Model file for the job. Use its own axes, mm. A direction names the side the tool comes from. Round coordinates to 2 decimals unless told otherwise and drop trailing zeros. Loops run counter-clockwise (first coordinate to the right, second up) from the corner with the lowest first, then second, coordinate; pieces in that order, holes last. Notation, with made-up numbers: M 80.25,0 L 92.25,0 A29 ccw 92.25,21 Z; hole C -37,56.5 d10. An arc over 180 degrees is marked long. Use a Markdown table: item, result. Add a question column.
Q1. Mould opens along Y. For faces 3 (the face through (0, 24.275, -7)), 4 (the face through (0.324, -4.697, -9.294)), 5 (the face through (0.185, -27.26, -5.297)) say: +Y half, -Y half, draft (parallel to the pull), parting line (faces both ways), or undercut.
Q2. Cut at B-B (z = -12). Give the cut face in (x, y), plus the area to 3 significant figures.
Q3. Probe line 1 (X direction, y = -27, z = -4.75); line 2 (Z direction, x = 0, y = -16.5); line 3 (Z direction, x = 1.25, y = -21). List the from-to ranges inside material, lowest first. Write a range as from..to.
Q4. Tool access for faces 1 (the face through (0.185, -1.711, -5.297)), 2 (the face through (0, -0.725, -6)): list every direction of +Z, -Z, +X, -X, +Y, -Y with a clear straight run to the whole face (end or side of a thin tool).
Q5. Pin check, flat tips, straight feed: pin 1 (3 mm diameter, centred on y = -17, z = -7, fed in from +X); pin 2 (5 mm diameter, centred on x = -5.5, y = -14, fed in from +Z); pin 3 (6 mm diameter, centred on y = -1.5, z = -4.5, fed in from -X); pin 4 (4.5 mm diameter, centred on x = 0, z = -3, fed in from -Y). Stop position of each tip, or through.
from build123d import *

# Parameters (mm, degrees)
REVOLVE1_ANGLE = 178.5


with BuildPart() as part:
    # Sketch1 → Revolve1 (revolve)
    with BuildSketch(Plane.XY):
        Polygon((5.3, 21.274776409), (5.3, 24.274776409), (13.3, 24.274776409), (13.3, -29.725223591), (5.3, -29.725223591), (5.3, -26.725223591), (5.3, -24.725223591), (9.3, -24.725223591), (9.3, -20.725223591), (5.3, -20.725223591), (5.3, -18.725223591), (9.3, -18.725223591), (9.3, -14.725223591), (5.3, -14.725223591), (5.3, -12.725223591), (9.3, -12.725223591), (9.3, -8.725223591), (5.3, -8.725223591), (5.3, -6.725223591), (9.3, -6.725223591), (9.3, -2.725223591), (5.3, -2.725223591), (5.3, -0.725223591), (9.3, -0.725223591), (9.3, 3.274776409), (5.3, 3.274776409), (5.3, 5.274776409), (9.3, 5.274776409), (9.3, 9.274776409), (5.3, 9.274776409), (5.3, 11.274776409), (9.3, 11.274776409), (9.3, 15.274776409), (5.3, 15.274776409), (5.3, 17.274776409), (9.3, 17.274776409), (9.3, 21.274776409), align=None)
    revolve(axis=Axis((0, -24, 0), (0, 1, 0)), revolution_arc=REVOLVE1_ANGLE)


solid = part.part
Checked values:
| question | item | result |
|---|---|---|
| 1 | face 3 | +Y half |
| 1 | face 4 | undercut |
| 1 | face 5 | draft |
| 2 | outline | M -5.73,-29.73 L 5.73,-29.73 L 5.73,24.27 L -5.73,24.27 Z |
| 2 | area | 619 mm^2 |
| 3 | line 1 | x = -12.42..-2.35, 2.35..12.42 |
| 3 | line 2 | z = -13.3..-9.3 |
| 3 | line 3 | z = -13.24..-9.22 |
| 4 | face 1 | +Z, +Y, -Y |
| 4 | face 2 | +Z |
| 5 | pin 1 | stops at x = 12.11 |
| 5 | pin 2 | stops at z = -0.14 |
| 5 | pin 3 | stops at x = -13.22 |
| 5 | pin 4 | passes through |
